```python
from build123d import *

# Parameters (mm, degrees)
SKETCH_1_R                   = 5
EXTRUDE_1_DEPTH              = 2
SKETCH_2_R                   = 6
EXTRUDE_2_DEPTH              = 2
HOLE_WIZARD_M4_1_D           = 4.5
HOLE_WIZARD_M4_1_CBORE_D     = 8
HOLE_WIZARD_M4_1_CBORE_DEPTH = 2


with BuildPart() as part:
    # 스케치1 → 보스-돌출1 (new body)
    with BuildSketch(Plane(origin=(0, 0, 0), x_dir=(1, 0, 0), z_dir=(0, 1, 0))):
        Circle(SKETCH_1_R)
    extrude(amount=EXTRUDE_1_DEPTH)

    # 스케치2 → 보스-돌출2 (add)
    with BuildSketch(Plane(origin=(0, 2, 0), x_dir=(1, 0, 0), z_dir=(0, 1, 0))):
        Circle(SKETCH_2_R)
    extrude(amount=EXTRUDE_2_DEPTH)

    # M4 육각 소켓 머리 캡 나사용 카운터보어1 (through all)
    with Locations(Plane(origin=(0, 4, 0), x_dir=(1, 0, 0), z_dir=(0, 1, 0))):
        with Locations((0, 0)):
            CounterBoreHole(HOLE_WIZARD_M4_1_D / 2, HOLE_WIZARD_M4_1_CBORE_D / 2, HOLE_WIZARD_M4_1_CBORE_DEPTH)


solid = part.part
```
Can you work these out from the model? Positions are in its coordinate system, mm. A direction names the side the tool comes from. Round coordinates to 2 decimals unless told otherwise and drop trailing zeros. Order: outer loops, then holes, each group sorted by start corner. A loop starts at its lowest first (then second) coordinate and runs counter-clockwise, first axis right, second up.
(1) We'd pull the mould along X, two halves only. Please class faces 4 (the face through (-1.42, 4, 3.92)), 5 (the face through (-6, 3, 0)), 6 (the face through (2, 2, 2)): +X half, -X half, draft (parallel to the pull), parting line (faces both ways), or undercut.
Results are:
face 4: draft
face 5: parting line
face 6: undercut
(2) If we section it at B-B (x = 0): Please give me the cut outline in (y, z), plus the area to 3 significant figures.
Results are:
outline: (0, -5) - (2, -5) - (2, -6) - (4, -6) - (4, -4) - (2, -4) - (2, -2.25) - (0, -2.25) - close; (0, 2.25) - (2, 2.25) - (2, 4) - (4, 4) - (4, 6) - (2, 6) - (2, 5) - (0, 5) - close
area: 19.0 mm2
(3) If we section it at C-C (y = 0.55): Please give me the cut outline in (x, z).
Results are:
outline: circle Ø10 at (0, 0); hole circle Ø4.5 at (0, 0)
(4) If I drill on L1, parallel to Z at x = 0, y = 0.7; L2, parallel to Z at x = 0, y = 2.9; L3, parallel to Y at x = -2.5, z = -0.25, over which ranges is the centre line in solid material (lowest first)?
Results are:
L1: z = -5 to -2.25, 2.25 to 5
L2: z = -6 to -4, 4 to 6
L3: y = 0 to 2
(5) If we section it at D-D (z = 4.75): Please give me the cut outline in (x, y), plus the area to 3 significant figures.
Results are:
outline: (-3.67, 2) - (-1.56, 2) - (-1.56, 0) - (1.56, 0) - (1.56, 2) - (3.67, 2) - (3.67, 4) - (-3.67, 4) - close
area: 20.9 mm2
(6) If we section it at A-A (z = 0): Please give me the cut outline in (x, y), plus the area to 3 significant figures.
Results are:
outline: (-6, 2) - (-5, 2) - (-5, 0) - (-2.25, 0) - (-2.25, 2) - (-4, 2) - (-4, 4) - (-6, 4) - close; (2.25, 0) - (5, 0) - (5, 2) - (6, 2) - (6, 4) - (4, 4) - (4, 2) - (2.25, 2) - close
area: 19.0 mm2
(7) I'm going to push flat-ended pins straight in: pin 1 (2.5 mm diameter, centred on x = 0, z = 0, fed in from -Y); pin 2 (5 mm diameter, centred on x = 0, z = 0, fed in from +Y); pin 3 (1 mm diameter, centred on x = -4.5, y = 3.5, fed in from +Z). Where does each tip first touch, or does it pass through?
Results are:
pin 1: passes through
pin 2: stops at y = 2
pin 3: stops at z = 4.47
(8) On a 3-axis mill with a long thin cutter (end or side, diameter ignored), from which of +Z, -Z, +X, -X, +Y, -Y can I reach the whole of each face in a straight line? I mean faces 1 (the face through (0.29, 0.99, -2.23)), 2 (the face through (-1.08, 0.99, 4.88)), 3 (the face through (-0.867, 3.014, 3.905)). Say none if no direction works.
Results are:
face 1: +Y, -Y
face 2: -Y
face 3: +Y
